Can you work these out from the model? Positions are in its coordinate system, mm. Face numbers are marked on the shaded views. A direction names the side the tool comes from. Coordinates: 2 decimals unless noted, no trailing zeros.
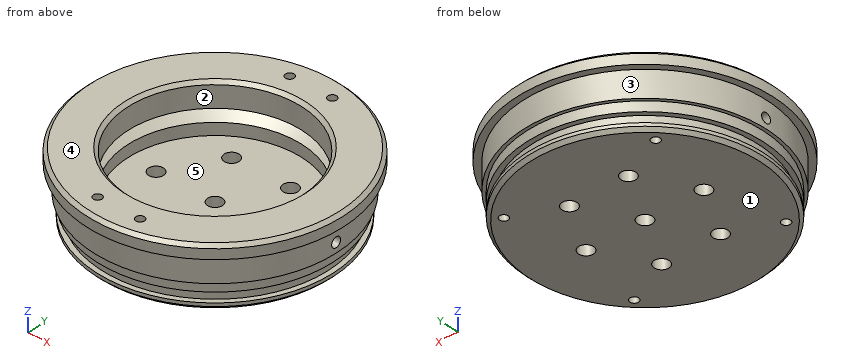
```python
from build123d import *

# Parameters (mm, degrees)
SKETCH_1_R               = 39
EXTRUDE_1_DEPTH          = 4
SKETCH_3_R               = 37
EXTRUDE_2_DEPTH          = 8
SKETCH_4_R               = 36
EXTRUDE_3_DEPTH          = 8
SKETCH_5_W               = 3
SKETCH_5_H               = 1.5
SKETCH_7_R               = 27
CUT_EXTRUDE_1_DEPTH      = 17
CHAMFER_2_SIZE           = 1
SKETCH_18_R              = 1.3
CUT_EXTRUDE_6_DEPTH      = 7
EXTRUDE_START            = 17
SKETCH_19_R              = 27
EXTRUDE_4_DEPTH          = 17
SKETCH_20_R              = 26.5
CUT_EXTRUDE_7_DEPTH      = 15
SKETCH_21_R              = 2.25
CUT_EXTRUDE_8_DEPTH      = 15
SKETCH_23_R              = 1.3
CUT_EXTRUDE_9_DEPTH      = 7
CUT_EXTRUDE_START        = 38
SKETCH_25_R              = 1.5
CUT_EXTRUDE_11_DEPTH     = 4
PATTERN_CIRCULAR_2_COUNT = 2
CHAMFER_3_SIZE           = 1


with BuildPart() as part:
    # Sketch 1 → Бобышка-Вытянуть1 (new body)
    with BuildSketch(Plane.XY):
        Circle(SKETCH_1_R)
    extrude(amount=EXTRUDE_1_DEPTH)

    # Эскиз3 → Бобышка-Вытянуть2 (add)
    with BuildSketch(Plane(origin=(0, 0, 0), x_dir=(-1, 0, 0), z_dir=(0, 0, -1))):
        with Locations(Location((0, 0, 0), (0, 0, 180))):
            Circle(SKETCH_3_R)
    extrude(amount=EXTRUDE_2_DEPTH)

    # Эскиз4 → Бобышка-Вытянуть3 (add)
    with BuildSketch(Plane(origin=(0, 0, -8), x_dir=(-1, 0, 0), z_dir=(0, 0, -1))):
        Circle(SKETCH_4_R)
    extrude(amount=EXTRUDE_3_DEPTH)

    # Эскиз5 → Вырез-Повернуть1 (revolve, cut)
    with BuildSketch(Plane(origin=(0, 0, 0), x_dir=(0, 0, -1), z_dir=(1, 0, 0)), mode=Mode.PRIVATE) as cut_revolve_1_sk:
        with Locations((12.5, 35.25)):
            Rectangle(SKETCH_5_W, SKETCH_5_H)
    revolve(cut_revolve_1_sk.sketch.rotate(Axis((0, 0, 46.650977883), (0, 0, -1)), 90), axis=Axis((0, 0, 46.650977883), (0, 0, -1)), mode=Mode.SUBTRACT)

    # Эскиз7 → Вырез-Вытянуть1 (cut)
    with BuildSketch(Plane(origin=(0, 0, -16), x_dir=(-1, 0, 0), z_dir=(0, 0, -1))):
        Circle(SKETCH_7_R)
    extrude(amount=-CUT_EXTRUDE_1_DEPTH, mode=Mode.SUBTRACT)

    # Фаска2
    chamfer_2_edges = [part.edges().sort_by_distance(p)[0] for p in [
        (36, 0, -16),
    ]]
    chamfer(chamfer_2_edges, length=CHAMFER_2_SIZE)

    # Эскиз18 → Вырез-Вытянуть6 (cut)
    with BuildSketch(Plane.XY.offset(4)):
        with Locations((6.5, 32.5)):
            Circle(SKETCH_18_R)
        with Locations(Location((-6.5, 32.5, 0), (0, 0, 180))):
            Circle(SKETCH_18_R)
        with Locations(Location((6.5, -32.5, 0), (0, 0, 180))):
            Circle(SKETCH_18_R)
        with Locations((-6.5, -32.5)):
            Circle(SKETCH_18_R)
    extrude(amount=-CUT_EXTRUDE_6_DEPTH, mode=Mode.SUBTRACT)

    # Эскиз19 → Бобышка-Вытянуть4 (add)
    with BuildSketch(Plane(origin=(0, 0, 1), x_dir=(-1, 0, 0), z_dir=(0, 0, -1)).offset(EXTRUDE_START)):
        Circle(SKETCH_19_R)
    extrude(amount=-EXTRUDE_4_DEPTH)

    # Эскиз20 → Вырез-Вытянуть7 (cut)
    with BuildSketch(Plane.XY.offset(4)):
        Circle(SKETCH_20_R)
    extrude(amount=-CUT_EXTRUDE_7_DEPTH, mode=Mode.SUBTRACT)

    # Эскиз21 → Вырез-Вытянуть8 (cut)
    with BuildSketch(Plane.XY.offset(-11)):
        with Locations((-18, 0)):
            Circle(SKETCH_21_R)
        with Locations((-9, 15.588457268)):
            Circle(SKETCH_21_R)
        with Locations((9, 15.588457268)):
            Circle(SKETCH_21_R)
        with Locations((18, 0)):
            Circle(SKETCH_21_R)
        with Locations((9, -15.588457268)):
            Circle(SKETCH_21_R)
        with Locations((-9, -15.588457268)):
            Circle(SKETCH_21_R)
        Circle(SKETCH_21_R)
    extrude(amount=-CUT_EXTRUDE_8_DEPTH, mode=Mode.SUBTRACT)

    # Эскиз22 → Вырез-Повернуть2 (revolve, cut)
    with BuildSketch(Plane(origin=(0, 0, 0), x_dir=(0, 0, -1), z_dir=(1, 0, 0)), mode=Mode.PRIVATE) as cut_revolve_2_sk:
        Polygon((3.5, 26.5), (5.383390473, 29.817478189), (7.363463637, 26.5), align=None)
    revolve(cut_revolve_2_sk.sketch.rotate(Axis((0, 0, 32.005569053), (0, 0, -1)), 90), axis=Axis((0, 0, 32.005569053), (0, 0, -1)), mode=Mode.SUBTRACT)

    # Эскиз23 → Вырез-Вытянуть9 (cut)
    with BuildSketch(Plane(origin=(0, 0, -16), x_dir=(-1, 0, 0), z_dir=(0, 0, -1))):
        with Locations((23.180408503, 22.060568026)):
            Circle(SKETCH_23_R)
        with Locations(Location((-23.180408503, 22.060568026, 0), (0, 0, 180))):
            Circle(SKETCH_23_R)
        with Locations(Location((23.180408503, -22.060568026, 0), (0, 0, 180))):
            Circle(SKETCH_23_R)
        with Locations((-23.180408503, -22.060568026)):
            Circle(SKETCH_23_R)
    extrude(amount=-CUT_EXTRUDE_9_DEPTH, mode=Mode.SUBTRACT)

    # Эскиз25 → Вырез-Вытянуть11 (cut)
    with BuildSketch(Plane(origin=(0, 0, 0), x_dir=(0, 0, -1), z_dir=(1, 0, 0)).offset(CUT_EXTRUDE_START)):
        with Locations((5, 0)):
            Circle(SKETCH_25_R)
    cut_extrude_11 = extrude(amount=-CUT_EXTRUDE_11_DEPTH, mode=Mode.SUBTRACT)

    # Круговой массив2: Вырез-Вытянуть11 ×2 about axis
    pattern_circular_2_axis = Axis((0, 0, -8), (0, 0, 1))
    for i in range(1, PATTERN_CIRCULAR_2_COUNT):
        add(cut_extrude_11.rotate(pattern_circular_2_axis, i * 360 / PATTERN_CIRCULAR_2_COUNT), mode=Mode.SUBTRACT)

    # Фаска3
    chamfer_3_edges = [part.edges().sort_by_distance(p)[0] for p in [
        (-39, 0, 4),
        (-26.5, 0, 4),
    ]]
    chamfer(chamfer_3_edges, length=CHAMFER_3_SIZE)


solid = part.part
```
Item 1: Suppose I cut it at A-A, the plane y = -16.5. Count the separate pieces of the cut face and the enclosed holes in it, plus the area to 3 significant figures.
Results are:
separate pieces: 3
enclosed holes: 0
area: 632 mm2
Item 2: On a 3-axis mill with a long thin cutter (end or side, diameter ignored), from which of +Z, -Z, +X, -X, +Y, -Y can I reach the whole of each face in a straight line? I mean the marked faces 1 and 2. Say none if no direction works.
Results are:
face 1: -Z, +X, -X, +Y, -Y
face 2: +Z
Item 3: I'm going to push flat-ended pins straight in: P1, Ø3, axis at y = -8.5, z = -7, coming from the -X side; P2, Ø4, axis at x = 0, y = 0, coming from the +Z side (1 decimal); P3, Ø3.5, axis at x = 23.18, y = -22.06, coming from the -Z side; P4, Ø6, axis at x = -28.5, z = -5, coming from the -Y side. Where does each tip first touch, or does it pass through?
Results are:
P1: stops at x = -36.33
P2: passes through
P3: stops at z = -16
P4: stops at y = -26.81
Item 4: I need wall thicknesses on line 1 along Y through (x, z) = (6.5, 1); line 2 along X through (y, z) = (0, -8.55); line 3 along X through (y, z) = (-22.5, -9.25). Which ranges of each line are inside material? Lowest first, please.
Results are:
line 1: y = -38.45 to -33.8, -31.2 to -25.69, 25.69 to 31.2, 33.8 to 38.45
line 2: x = -36 to -26.5, 26.5 to 36
line 3: x = -28.1 to -24.4, -21.96 to -14, 14 to 21.96, 24.4 to 28.1
Item 5: We'd pull the mould along X, two halves only. Please class the marked faces 3, 4 and 5: +X half, -X half, draft (parallel to the pull), parting line (faces both ways), or undercut.
Results are:
face 3: parting line
face 4: draft
face 5: undercut
